from build123d import *

# Parameters (mm, degrees)
F1_DEPTH = 25.4
F2_R     = 15.875
F3_DEPTH = 25.401


with BuildPart() as f1:
    # F0 (on Top) → F1 (new body)
    with BuildSketch(Plane.XY):
        with BuildLine():
            Line((353.500903, 182.437663), (-347.539097, 182.437663))
            Line((-347.539097, 182.437663), (-347.539097, 23.687663))
            Line((-347.539097, 23.687663), (-309.439097, 23.687663))
            ThreePointArc((-309.439097, 23.687663), (-303.089106, 17.348244), (-309.417936, 10.987698))
            ThreePointArc((-309.417936, 10.987698), (-309.439097, 10.987663), (-309.460259, 10.987698))
            Line((-309.460259, 10.987698), (-347.539097, 10.987698))
            Line((-347.539097, 10.987698), (-347.539097, -160.462337))
            Line((-347.539097, -160.462337), (353.500903, -160.462337))
            Line((353.500903, -160.462337), (353.500903, 182.437663))
        make_face()
        with BuildLine():
            ThreePointArc((204.910903, 10.987663), (198.560903, 17.337663), (204.910903, 23.687663))
            Line((204.910903, 23.687663), (281.110903, 23.687663))
            ThreePointArc((281.110903, 23.687663), (287.460903, 17.337663), (281.110903, 10.987663))
            Line((281.110903, 10.987663), (204.910903, 10.987663))
        make_face(mode=Mode.SUBTRACT)
    extrude(amount=F1_DEPTH)

    # F2 (on face) → F3 (cut, through all)
    with BuildSketch(Plane.XY.offset(25.4)):
        with Locations((-4.639097, -122.362337)):
            Circle(F2_R)
    extrude(amount=-F3_DEPTH, mode=Mode.SUBTRACT)


solid = f1.part
Build history of the part. All positions in model axes, mm. A direction names the side the tool comes from. Give positions to 0.01 mm unless a question says otherwise; leave off trailing zeros. Order: outer loops, then holes, each group sorted by start corner. A loop starts at its lowest first (then second) coordinate and runs counter-clockwise, first axis right, second up. Notation, with made-up numbers: M 57.25,24.5 L 65.25,24.5 A12 ccw 65.25,28.5 Z; hole C 8,28.25 d10. An arc over 180 degrees is marked long. Put each result on its own line as item: value.
Item 1: Probe line 1 (Y direction, x = 204, z = 14.5); line 2 (Y direction, x = 244.5, z = 11.5); line 3 (X direction, y = -125, z = 10). List the from-to ranges inside material, lowest first. Write a range as [from, to].
From the geometry:
line 1: y = [-160.46, 11.05], [23.62, 182.44]
line 2: y = [-160.46, 10.99], [23.69, 182.44]
line 3: x = [-347.54, -20.29], [11.02, 353.5]
Item 2: Slice it at B-B, the plane x = 1. Write the cut outline in (y, z), plus the area to 3 significant figures.
From the geometry:
outline: M -160.46,0 L -137.2,0 L -137.2,25.4 L -160.46,25.4 Z; M -107.52,0 L 182.44,0 L 182.44,25.4 L -107.52,25.4 Z
area: 7,960 mm2
Item 3: Two-plate mould, pull along X, no slides. Class faces 1 (the flat face through (-329, 23.688, 13)), 2 (the flat face through (244, 10.988, 13)), 3 (the flat face through (-347.539, 104, 13)): +X half, -X half, draft (parallel to the pull), parting line (faces both ways), or undercut.
From the geometry:
face 1: draft
face 2: undercut
face 3: -X half
Item 4: Slice it at A-A, the plane x = 265.5. Write the cut outline in (y, z).
From the geometry:
outline: M -160.46,0 L 10.99,0 L 10.99,25.4 L -160.46,25.4 Z; M 23.69,0 L 182.44,0 L 182.44,25.4 L 23.69,25.4 Z
Item 5: 3-axis set-ups, long thin cutter, end or side, ignore diameter. For faces 4 (the flat face through (-328, 10.988, 13)), 5 (the flat face through (8, 182.438, 13)), 6 (the cylindrical face through (198.562, 17.198, 12.522)): which of +Z, -Z, +X, -X, +Y, -Y reach the whole face in a straight line?
From the geometry:
face 4: +Z, -Z, -X
face 5: +Z, -Z, +X, -X, +Y
face 6: +Z, -Z
